from build123d import *

# Parameters (mm, degrees)
EXTRUDE_1_DEPTH     = 20
EXTRUDE_1_2_DEPTH   = 10
CHAMFER_1_SIZE      = 6
CHAMFER_2_SIZE      = 1
CUT_EXTRUDE_1_REACH = 74.497
SKETCH_3_W          = 6
SKETCH_3_H          = 20
CUT_EXTRUDE_2_REACH = 79.965
SKETCH_4_W          = 6
SKETCH_4_H          = 20
FILLET_1_R          = 10
FILLET_2_R          = 2
FILLET_3_R          = 1


with BuildPart() as part:
    # Эскиз1 → Extrude 1 (new body)
    with BuildSketch(Plane(origin=(0, 0, 0), x_dir=(1, 0, 0), z_dir=(0, 1, 0))):
        Polygon((1.2, -1.2), (-47.8, -1.2), (-47.8, -41.2), (-56.2, -41.2), (-56.2, 10.2), (-47.8, 10.2), (-47.8, 7.2), (1.2, 7.2), align=None)
        Polygon((0, 0), (-49, 0), (-49, -40), (-55, -40), (-55, 9), (-49, 9), (-49, 6), (0, 6), align=None, mode=Mode.SUBTRACT)
    extrude(amount=EXTRUDE_1_DEPTH)

    # Эскиз2 → Extrude 1 2 (add)
    with BuildSketch(Plane.XZ):
        Polygon((-56.2, 41.2), (-47.8, 41.2), (-47.8, 1.2), (1.2, 1.2), (1.2, -7.2), (-47.8, -7.2), (-47.8, -10.2), (-56.2, -10.2), align=None)
    extrude(amount=EXTRUDE_1_2_DEPTH)

    # Фаска1
    chamfer_1_edges = [part.edges().sort_by_distance(p)[0] for p in [
        (1.2, -10, -3),
    ]]
    chamfer(chamfer_1_edges, length=CHAMFER_1_SIZE)
    chamfer_1_2_edges = [part.edges().sort_by_distance(p)[0] for p in [
        (-52, -10, -10.2),
    ]]
    chamfer(chamfer_1_2_edges, length=CHAMFER_1_SIZE)
    chamfer_1_3_edges = [part.edges().sort_by_distance(p)[0] for p in [
        (-52, -10, 41.2),
    ]]
    chamfer(chamfer_1_3_edges, length=CHAMFER_1_SIZE)

    # Фаска2
    chamfer_2_edges = [part.edges().sort_by_distance(p)[0] for p in [
        (-47.8, -10, 18.2),
        (-56.2, -10, 15.5),
        (-26.3, -10, 1.2),
    ]]
    chamfer(chamfer_2_edges, length=CHAMFER_2_SIZE)

    # Эскиз3 → Вырез-Вытянуть1 (cut, up to next)
    with BuildSketch(Plane.ZY, mode=Mode.PRIVATE) as cut_extrude_1_sk1:
        with Locations((-3, 10)):
            Rectangle(SKETCH_3_W, SKETCH_3_H)
    cut_extrude_1_tool1 = extrude(cut_extrude_1_sk1.sketch, amount=-CUT_EXTRUDE_1_REACH, mode=Mode.PRIVATE) & part.part
    add(cut_extrude_1_tool1.solids().sort_by_distance((0, 10, -3))[0], mode=Mode.SUBTRACT)

    # Эскиз4 → Вырез-Вытянуть2 (cut, up to next)
    with BuildSketch(Plane(origin=(0, 0, 40), x_dir=(-1, 0, 0), z_dir=(0, 0, -1)), mode=Mode.PRIVATE) as cut_extrude_2_sk1:
        with Locations((52, 10)):
            Rectangle(SKETCH_4_W, SKETCH_4_H)
    cut_extrude_2_tool1 = extrude(cut_extrude_2_sk1.sketch, amount=-CUT_EXTRUDE_2_REACH, mode=Mode.PRIVATE) & part.part
    add(cut_extrude_2_tool1.solids().sort_by_distance((-52, 10, 40))[0], mode=Mode.SUBTRACT)

    # Скругление1
    fillet_1_edges = [part.edges().sort_by_distance(p)[0] for p in [
        (1.2, 20, -6.6),
        (-48.4, 20, 41.2),
        (-55.6, 20, 41.2),
        (1.2, 20, 0.6),
    ]]
    fillet(fillet_1_edges, radius=FILLET_1_R)

    # Скругление2
    fillet_2_edges = [part.edges().sort_by_distance(p)[0] for p in [
        (-47.8, 5.5, 1.2),
        (-47.8, 6.5, -7.2),
    ]]
    fillet(fillet_2_edges, radius=FILLET_2_R)

    # Скругление3
    fillet_3_edges = [part.edges().sort_by_distance(p)[0] for p in [
        (-56.2, 8, -10.2),
        (-47.8, 8, -10.2),
        (-49, 10, -6),
        (-49, 10, 0),
    ]]
    fillet(fillet_3_edges, radius=FILLET_3_R - 0.0001)  # a hair under: the kernel refuses the full size


solid = part.part
For this review, take the finished solid that the model builds, in its own axes (mm). A direction names the side the tool comes from. Coordinates: 2 decimals unless noted, no trailing zeros. Order: outer loops, then holes, each group sorted by start corner. A loop starts at its lowest first (then second) coordinate and runs counter-clockwise, first axis right, second up. Notation, with made-up numbers: (-31.5, 28) - (-24.5, 28) arc R15 ccw to (-24.5, 50) - close; hole circle Ø3 at (50.5, 88.5). An arc over 180 degrees is marked (long way). Answer as CSV lines item,"result". Start each with the question number.
1) Draft analysis for pull direction Z (two halves, no side actions). For faces 1 (the flat face through (-26.6, -9.4, 0.8)), 2 (the flat face through (-38, 20, 1)), 3 (the flat face through (-24, 10, 0)), state which applies: +Z half, -Z half, draft (parallel to the pull), parting line (faces both ways), or undercut.
2) Add section C-C (x = -52). State the section outline as (y, z) points, then the cut area to 3 significant figures.
3) Insertion check: P1, Ø8, axis at y = 16, z = 9.5, coming from the +X side; P2, Ø8, axis at x = -36, y = -3, coming from the +Z side; P3, Ø6, axis at x = -24.5, z = 6.5, coming from the -Y side; P4, Ø8, axis at x = -27.5, y = 0.5, coming from the -Z side. Each pin has a flat end and moves straight along its axis. Give the tip position at first contact, or say it passes through.
4) Machinability: for faces 4 (the flat face through (-37, 0, -1)), 5 (the flat face through (-48.2, -9.4, 18.5)), 6 (the flat face through (-22, 7, -7.2)), 7 (the flat face through (-49, 10, -8)), 8 (the flat face through (-24, 10, -6)), which of the approach directions +Z, -Z, +X, -X, +Y, -Y give a long, thin tool a straight path to every point of the face, cutting with its end or side? Answer none if there is none.
5) Add section B-B (z = -3). State the section outline as (x, y) points.
6) To check wall thickness, follow line 1 along X through (y, z) = (8, 1); line 2 along X through (y, z) = (13.5, 21); line 3 along Z through (x, y) = (-6.5, 5.5). State the ranges of each line that lie inside material, in increasing order. Write a range as [from, to].
Result:
1,face 1,"+Z half"
1,face 2,"draft"
1,face 3,"undercut"
2,outline,"(-10, -4.2) - (-4, -10.2) - (20, -10.2) - (20, -9) - (0, -9) - (0, 41.2) - (-4, 41.2) - (-10, 35.2) - close"
2,area,"502 mm^2"
3,P1,"x = -47.8"
3,P2,"z = 1.2"
3,P3,"through"
3,P4,"z = -7.2"
4,face 4,"+Y"
4,face 5,"+Z, +X, -Y"
4,face 6,"-Z, +X, +Y, -Y"
4,face 7,"+Z, +Y"
4,face 8,"+X, +Y"
5,outline,"(-56.2, -9) - (-55.2, -10) - (-4.8, -10) - (1.2, -4) - (1.2, 0) - (-55, 0) - (-55, 20) - (-56.2, 20) - close"
6,line 1,"[-56.2, -55], [-49, 1.2]"
6,line 2,"[-56.2, -55], [-49, -47.8]"
6,line 3,"[-7.2, -6], [0, 1.2]"
